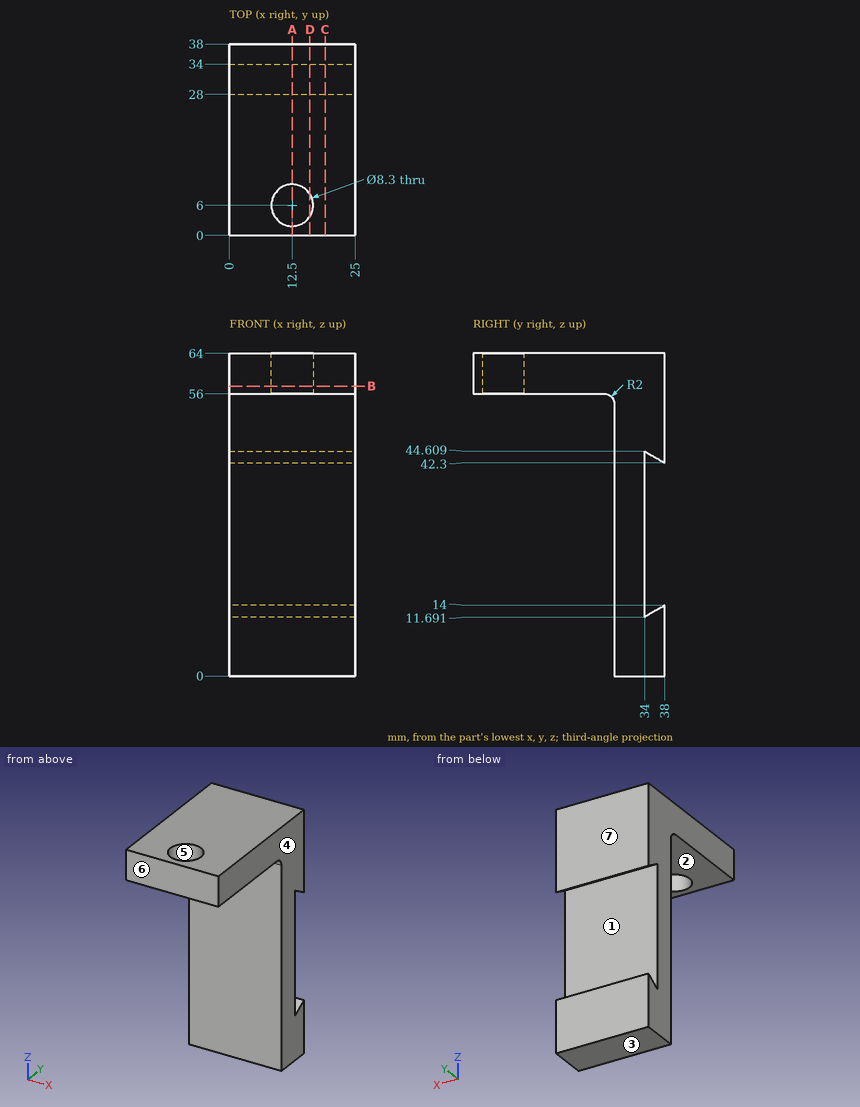
Input: dimensioned drawing with shaded views. Units: mm. Origin: part minimum x, y, z. A direction names the side the tool comes from. Coordinates: 2 decimals unless noted, no trailing zeros. Order: outer loops, then holes, each group sorted by start corner. A loop starts at its lowest first (then second) coordinate and runs counter-clockwise, first axis right, second up.
1. Cut plane C-C, the plane x = 19. Return loops of the section in (y, z).
Checked values:
outline: (0, 56) - (26, 56) arc R2 cw to (28, 54) - (28, 0) - (38, 0) - (38, 14) - (34, 11.69) - (34, 44.61) - (38, 42.3) - (38, 64) - (0, 64) - close
2. Ray query, line 1 along Y through (x, z) = (12.5, 58.25); line 2 along Z through (x, y) = (14.5, 19); line 3 along Y through (x, z) = (9.5, 5.5). Return the intervals inside material, ascending.
Checked values:
line 1: y = 0 to 1.85, 10.15 to 38
line 2: z = 56 to 64
line 3: y = 28 to 38
3. Cut plane D-D, the plane x = 16. Return loops of the section in (y, z), plus the area to 3 significant figures.
Checked values:
outline: (0, 56) - (3.77, 56) - (3.77, 64) - (0, 64) - close; (8.23, 56) - (26, 56) arc R2 cw to (28, 54) - (28, 0) - (38, 0) - (38, 14) - (34, 11.69) - (34, 44.61) - (38, 42.3) - (38, 64) - (8.23, 64) - close
area: 707 mm2
4. Draft query along Y for the marked faces 4, 5, 6 and 7. Return one class per face: +Y half, -Y half, draft (parallel to the pull), parting line (faces both ways), or undercut.
Checked values:
face 4: draft
face 5: undercut
face 6: -Y half
face 7: +Y half
5. Cut plane A-A, the plane x = 12.5. Return loops of the section in (y, z), plus the area to 3 significant figures.
Checked values:
outline: (0, 56) - (1.85, 56) - (1.85, 64) - (0, 64) - close; (10.15, 56) - (26, 56) arc R2 cw to (28, 54) - (28, 0) - (38, 0) - (38, 14) - (34, 11.69) - (34, 44.61) - (38, 42.3) - (38, 64) - (10.15, 64) - close
area: 676 mm2
6. Contact query for flat-ended pins moving along their axis: P1, Ø11, axis at x = 12.5, y = 6, coming from the +Z side; P2, Ø12.5, axis at x = 16, z = 30, coming from the +Y side; P3, Ø12.5, axis at x = 12.5, y = 10.5, coming from the -Z side; P4, Ø1.5, axis at x = 6, z = 9.5, coming from the -Y side. Output: stop coordinate, or through.
Checked values:
P1: stops at z = 64
P2: stops at y = 34
P3: stops at z = 56
P4: stops at y = 28
7. Cut plane B-B, the plane z = 57.5. Return loops of the section in (x, y), plus the area to 3 significant figures.
Checked values:
outline: (0, 0) - (25, 0) - (25, 38) - (0, 38) - close; hole circle Ø8.3 at (12.5, 6)
area: 896 mm2
8. Access query for the marked faces 1, 2 and 3. Directions: +Z, -Z, +X, -X, +Y, -Y. A direction counts if a zero-diameter tool reaches every point of the face in a straight line with its end or side. Return the directions, or none.
Checked values:
face 1: +X, -X
face 2: -Z, +X, -X, -Y
face 3: -Z, +X, -X, +Y, -Y
